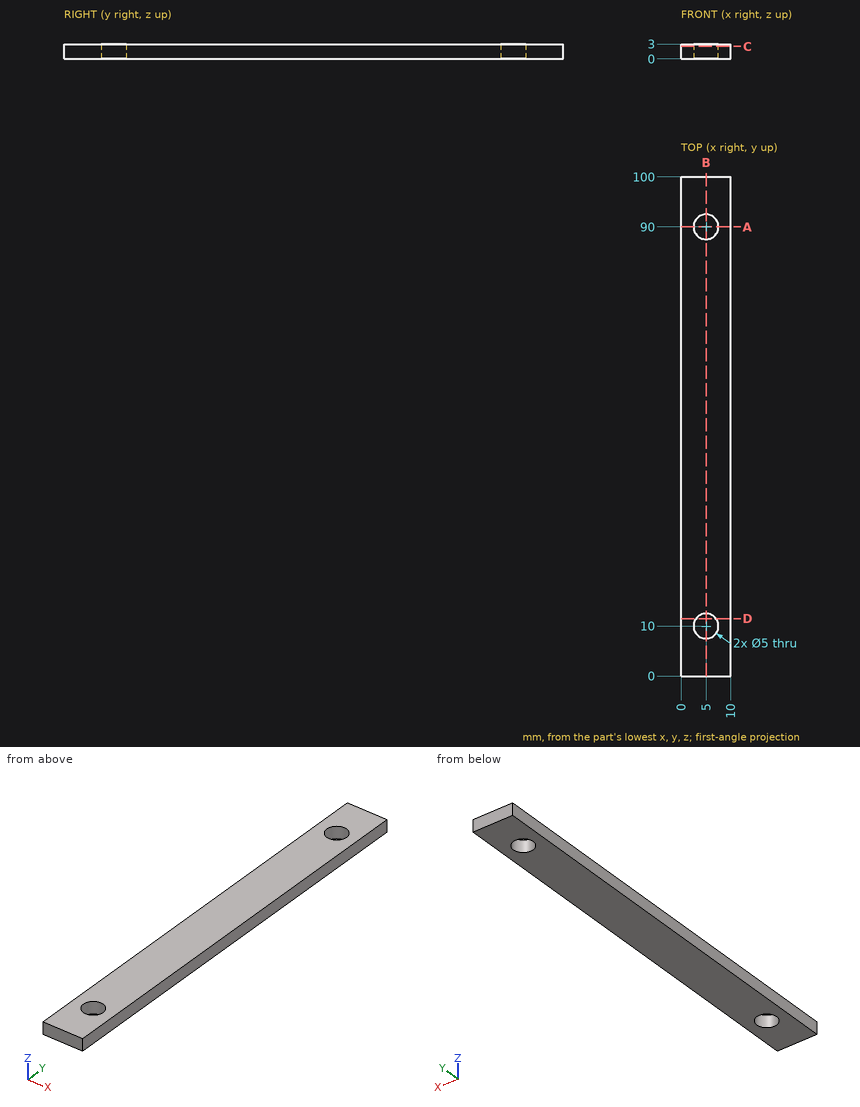
Print and shaded views of the part. All mm, measured from the part's lowest x, y and z. Coordinates: 2 decimals unless noted, no trailing zeros. Loops run counter-clockwise (first coordinate to the right, second up) from the corner with the lowest first, then second, coordinate; pieces in that order, holes last. Notation, with made-up numbers: (-22, 49) -> (-15, 49) arc R20 ccw to (-15, 68) -> close; hole circle Ø1 at (14.25, 83.5). An arc over 180 degrees is marked (long way). Use a Markdown table: item, result. Add a question column.
Item 1: Probe probe 1 along Y at (x, z) = (5, 1.4); probe 2 along Y at (x, z) = (2.75, 1.75). List the from-to ranges inside material, lowest first.
Item 2: Flat gauge pin, fed straight in: P1, Ø4, axis at x = 5, y = 10, coming from the -Z side. Where does the tip first touch, or does it go through?
Item 3: Band-saw the part on A-A on y = 90. Write the cut outline in (x, z), plus the area to 3 significant figures.
Item 4: Band-saw the part on B-B on x = 5. Write the cut outline in (y, z), plus the area to 3 significant figures.
Item 5: Band-saw the part on D-D on y = 11.5. Write the cut outline in (x, z).
Item 6: Band-saw the part on C-C on z = 2.5. Write the cut outline in (x, y), plus the area to 3 significant figures.
Geometry says:
| question | item | result |
|---|---|---|
| 1 | probe 1 | 0 to 7.5, 12.5 to 87.5, 92.5 to 100 |
| 1 | probe 2 | 0 to 8.91, 11.09 to 88.91, 91.09 to 100 |
| 2 | P1 | through |
| 3 | outline | (0, 0) -> (2.5, 0) -> (2.5, 3) -> (0, 3) -> close; (7.5, 0) -> (10, 0) -> (10, 3) -> (7.5, 3) -> close |
| 3 | area | 15.0 mm² |
| 4 | outline | (0, 0) -> (7.5, 0) -> (7.5, 3) -> (0, 3) -> close; (12.5, 0) -> (87.5, 0) -> (87.5, 3) -> (12.5, 3) -> close; (92.5, 0) -> (100, 0) -> (100, 3) -> (92.5, 3) -> close |
| 4 | area | 270 mm² |
| 5 | outline | (0, 0) -> (3, 0) -> (3, 3) -> (0, 3) -> close; (7, 0) -> (10, 0) -> (10, 3) -> (7, 3) -> close |
| 6 | outline | (0, 0) -> (10, 0) -> (10, 100) -> (0, 100) -> close; hole circle Ø5 at (5, 10); hole circle Ø5 at (5, 90) |
| 6 | area | 961 mm² |
